Part model, mm, in its own coordinate system. A direction names the side the tool comes from. Give positions to 0.01 mm unless a question says otherwise; leave off trailing zeros. Order: outer loops, then holes, each group sorted by start corner. A loop starts at its lowest first (then second) coordinate and runs counter-clockwise, first axis right, second up. Notation, with made-up numbers: M 35,52.25 L 77,52.25 A23 ccw 77,60.25 Z; hole C 20,53 d4. An arc over 180 degrees is marked long. Answer as a JSON object with one key per item and string values.
from build123d import *

# Parameters (mm, degrees)
F0_W     = 19.05
F0_H     = 76.2
F1_DEPTH = 12.7
F3_DEPTH = 38.1
F4_W     = 15.875
F4_H     = 6.35
F5_DEPTH = 19.051
F6_R     = 2.5
F7_DEPTH = 12.701


with BuildPart() as f1:
    # F0 (on Top) → F1 (new body)
    with BuildSketch(Plane.XY):
        Rectangle(F0_W, F0_H)
    extrude(amount=F1_DEPTH)

    # F2 (on face) → F3 (join)
    with BuildSketch(Plane.XY.offset(12.7)):
        with BuildLine():
            Line((-9.525, -38.1), (9.525, -38.1))
            ThreePointArc((9.525, -38.1), (0, -28.575), (-9.525, -38.1))
        make_face()
    extrude(amount=F3_DEPTH)

    # F4 (on face) → F5 (cut, through all)
    with BuildSketch(Plane(origin=(-9.525, 0, 0), x_dir=(0, -1, 0), z_dir=(-1, 0, 0))):
        with Locations((0, 12.7)):
            Rectangle(F4_W, F4_H)
    extrude(amount=-F5_DEPTH, mode=Mode.SUBTRACT)

    # F6 (on face) → F7 (cut, through all)
    with BuildSketch(Plane.XY.offset(12.7)):
        with Locations((0, -19.05)):
            Circle(F6_R)
        with Locations((0, 19.05)):
            Circle(F6_R)
    extrude(amount=-F7_DEPTH, mode=Mode.SUBTRACT)


solid = f1.part
1. Pin check, flat tips, straight feed: P1, Ø10, axis at x = 6, y = 10, coming from the +Z side; P2, Ø4, axis at x = -5, y = 1, coming from the -Z side; P3, Ø8, axis at x = 0.5, y = 0.5, coming from the +Z side (3 decimals); P4, Ø1, axis at x = 3, z = 41.5, coming from the +Y side. Stop position of each tip, or through.
Worked answers:
{"P1": "stops at z = 12.7", "P2": "stops at z = 0", "P3": "stops at z = 9.525", "P4": "stops at y = -28.91"}
2. Which spindle directions (+Z, -Z, +X, -X, +Y, -Y) get a long thin tool onto all of the face, cutting with end or side? Do faces 1 (the flat face through (0, -34, 50.8)), 2 (the flat face through (-9.525, -1, 6)), 3 (the cylindrical face through (0.209, -28.577, 31.483)), 4 (the flat face through (0, -7.938, 11)), 5 (the flat face through (0, 23, 12.7)). Say none if no direction does.
Worked answers:
{"face 1": "+Z, +X, -X, +Y, -Y", "face 2": "+Z, -Z, -X, +Y, -Y", "face 3": "+Z, +Y", "face 4": "+Z, +X, -X", "face 5": "+Z, +X, -X, +Y"}
3. Probe line 1 along Y through (x, z) = (0, 6.5); line 2 along Y through (x, z) = (0, 10); line 3 along Y through (x, z) = (5, 10). List the from-to ranges inside material, lowest first.
Worked answers:
{"line 1": "y = -38.1 to -21.55, -16.55 to 16.55, 21.55 to 38.1", "line 2": "y = -38.1 to -21.55, -16.55 to -7.94, 7.94 to 16.55, 21.55 to 38.1", "line 3": "y = -38.1 to -7.94, 7.94 to 38.1"}
4. Two-plate mould, pull along Y, no slides. Class faces 6 (the flat face through (9.525, -1, 6)), 7 (the flat face through (0, 0, 9.525)), 8 (the flat face through (0, 38.1, 6)), 9 (the cylindrical face through (1.15, 16.83, 6.44)): +Y half, -Y half, draft (parallel to the pull), parting line (faces both ways), or undercut.
Worked answers:
{"face 6": "draft", "face 7": "undercut", "face 8": "+Y half", "face 9": "undercut"}
5. Cut at B-B on y = -19.05. Give the cut face in (x, z) (3 decimals).
Worked answers:
{"outline": "M -9.525,0 L -2.5,0 L -2.5,12.7 L -9.525,12.7 Z; M 2.5,0 L 9.525,0 L 9.525,12.7 L 2.5,12.7 Z"}
6. Cut at C-C on z = 7.5. Give the cut face in (x, y) (3 decimals), plus the area to 3 significant figures.
Worked answers:
{"outline": "M -9.525,-38.1 L 9.525,-38.1 L 9.525,38.1 L -9.525,38.1 Z; hole C 0,-19.05 d5; hole C 0,19.05 d5", "area": "1,410 mm^2"}
7. Cut at A-A on x = 0. State how many separate pieces and enclosed holes the cut face has, plus the area to 3 significant figures.
Worked answers:
{"separate pieces": "3", "enclosed holes": "0", "area": "1,150 mm^2"}
8. Cut at D-D on x = 7.5. Give the cut face in (y, z) (1 decimal), plus the area to 3 significant figures.
Worked answers:
{"outline": "M -38.1,0 L 38.1,0 L 38.1,12.7 L 7.9,12.7 L 7.9,9.5 L -7.9,9.5 L -7.9,12.7 L -32.2,12.7 L -32.2,50.8 L -38.1,50.8 Z", "area": "1,140 mm^2"}
